```python
from build123d import *

# Parameters (mm, degrees)
SKETCH1_R           = 19.05
BOSS_EXTRUDE1_DEPTH = 76.2
SKETCH2_R           = 17.78
CUT_EXTRUDE1_DEPTH  = 69.85
CUT_EXTRUDE2_DEPTH  = 69.85
BOSS_EXTRUDE2_START = 6.35
SKETCH4_R           = 43.18
SKETCH4_R_2         = 17.78
BOSS_EXTRUDE2_DEPTH = 6.35
SKETCH5_R           = 12.7
BOSS_EXTRUDE3_DEPTH = 10.16
FILLET1_R           = 2.54
CHAMFER1_SIZE       = 2.54


with BuildPart() as part:
    # Sketch1 → Boss-Extrude1 (new body)
    with BuildSketch(Plane.XY):
        with Locations(Location((0, 0, 0), (0, 0, 180))):
            Circle(SKETCH1_R)
    extrude(amount=BOSS_EXTRUDE1_DEPTH)

    # Sketch2 → Cut-Extrude1 (cut)
    with BuildSketch(Plane.XY.offset(76.2)):
        Circle(SKETCH2_R)
    extrude(amount=-CUT_EXTRUDE1_DEPTH, mode=Mode.SUBTRACT)

    # Sketch3 → Cut-Extrude2 (cut)
    with BuildSketch(Plane.XY.offset(76.2)):
        with BuildLine():
            Line((-17.494221189, 3.175), (-18.783553311, 3.175))
            ThreePointArc((-18.783553311, 3.175), (-19.05, 0), (-18.783553311, -3.175))
            Line((-18.783553311, -3.175), (-17.494221189, -3.175))
            ThreePointArc((-17.494221189, -3.175), (-17.78, 0), (-17.494221189, 3.175))
        make_face()
        with BuildLine():
            ThreePointArc((19.05, 0), (18.983271459, 1.593080258), (18.783553311, 3.175))
            Line((18.783553311, 3.175), (17.494221189, 3.175))
            ThreePointArc((17.494221189, 3.175), (17.708411176, 1.593917699), (17.78, 0))
            ThreePointArc((17.78, 0), (17.708411176, -1.593917699), (17.494221189, -3.175))
            Line((17.494221189, -3.175), (18.783553311, -3.175))
            ThreePointArc((18.783553311, -3.175), (18.983271459, -1.593080258), (19.05, 0))
        make_face()
        with BuildLine():
            ThreePointArc((3.175, 18.783553311), (0, 19.05), (-3.175, 18.783553311))
            Line((-3.175, 18.783553311), (-3.175, 17.494221189))
            ThreePointArc((-3.175, 17.494221189), (0, 17.78), (3.175, 17.494221189))
            Line((3.175, 17.494221189), (3.175, 18.783553311))
        make_face()
        with BuildLine():
            Line((-3.175, -17.494221189), (-3.175, -18.783553311))
            ThreePointArc((-3.175, -18.783553311), (0, -19.05), (3.175, -18.783553311))
            Line((3.175, -18.783553311), (3.175, -17.494221189))
            ThreePointArc((3.175, -17.494221189), (0, -17.78), (-3.175, -17.494221189))
        make_face()
    extrude(amount=-CUT_EXTRUDE2_DEPTH, mode=Mode.SUBTRACT)

    # Sketch4 → Boss-Extrude2 (add)
    with BuildSketch(Plane.XY.offset(76.2).offset(BOSS_EXTRUDE2_START)):
        Circle(SKETCH4_R)
        Circle(SKETCH4_R_2, mode=Mode.SUBTRACT)
    extrude(amount=-BOSS_EXTRUDE2_DEPTH)

    # Sketch5 → Boss-Extrude3 (add)
    with BuildSketch(Plane(origin=(0, 0, 0), x_dir=(-1, 0, 0), z_dir=(0, 0, -1))):
        with Locations(Location((0, 0, 0), (0, 0, 180))):
            Circle(SKETCH5_R)
    extrude(amount=BOSS_EXTRUDE3_DEPTH)

    # Fillet1
    fillet1_edges = [part.edges().sort_by_distance(p)[0] for p in [
        (19.05, 0, 0),
        (-43.18, 0, 76.2),
        (-12.7, 0, -10.16),
    ]]
    fillet(fillet1_edges, radius=FILLET1_R)

    # Chamfer1
    # the kernel refuses this chamfer: 2.54 mm, written as the material it adds along each edge
    with BuildSketch(Plane(origin=(0, 0, 76.2), x_dir=(-0.9846344295499855, 0.1746282913641848, 0), z_dir=(0.1746282913641848, 0.9846344295499855, 0))) as chamfer1_piece_1_section:
        Polygon((19.05 + CHAMFER1_SIZE, 0), (19.05, -CHAMFER1_SIZE), (19.05, 0), align=None)
    chamfer1_piece_1 = revolve(axis=Axis((0, 0, 76.2), (0, 0, 1)), revolution_arc=110.114055389, mode=Mode.PRIVATE)
    chamfer1_piece_1 = split(chamfer1_piece_1, bisect_by=Plane(origin=(-19.847264072, 3.175, 75.490542074), z_dir=(0, 1, 0)), keep=Keep.TOP, mode=Mode.PRIVATE)
    add(chamfer1_piece_1)
    with BuildSketch(Plane(origin=(0, 0, 76.2), x_dir=(-0.9846344295499855, 0.1746282913641848, 0), z_dir=(0.1746282913641848, 0.9846344295499855, 0))) as chamfer1_piece_2_section:
        Polygon((19.05 + CHAMFER1_SIZE, 0), (19.05, -CHAMFER1_SIZE), (19.05, 0), align=None)
    chamfer1_piece_2 = revolve(axis=Axis((0, 0, 76.2), (0, 0, 1)), revolution_arc=110.114055389, mode=Mode.PRIVATE)
    chamfer1_piece_2 = split(chamfer1_piece_2, bisect_by=Plane(origin=(-14.346148442, -3.175, 74.961482306), z_dir=(0, -1, 0)), keep=Keep.TOP, mode=Mode.PRIVATE)
    chamfer1_piece_2 = split(chamfer1_piece_2, bisect_by=Plane(origin=(-3.175, -14.346148442, 74.961482306), z_dir=(-1, 0, 0)), keep=Keep.TOP, mode=Mode.PRIVATE)
    add(chamfer1_piece_2)
    with BuildSketch(Plane(origin=(0, 0, 76.2), x_dir=(-0.9846344295499855, 0.1746282913641848, 0), z_dir=(0.1746282913641848, 0.9846344295499855, 0))) as chamfer1_piece_3_section:
        Polygon((19.05 + CHAMFER1_SIZE, 0), (19.05, -CHAMFER1_SIZE), (19.05, 0), align=None)
    chamfer1_piece_3 = revolve(axis=Axis((0, 0, 76.2), (0, 0, 1)), revolution_arc=110.114055389, mode=Mode.PRIVATE)
    chamfer1_piece_3 = split(chamfer1_piece_3, bisect_by=Plane(origin=(3.175, -19.847263843, 75.490541907), z_dir=(1, 0, 0)), keep=Keep.TOP, mode=Mode.PRIVATE)
    add(chamfer1_piece_3)
    with BuildSketch(Plane(origin=(0, 0, 76.2), x_dir=(0.9846344295499821, -0.1746282913642033, 0), z_dir=(-0.1746282913642033, -0.9846344295499821, 0))) as chamfer1_piece_4_section:
        Polygon((19.05 + CHAMFER1_SIZE, 0), (19.05, -CHAMFER1_SIZE), (19.05, 0), align=None)
    chamfer1_piece_4 = revolve(axis=Axis((0, 0, 76.2), (0, 0, 1)), revolution_arc=110.114055389, mode=Mode.PRIVATE)
    chamfer1_piece_4 = split(chamfer1_piece_4, bisect_by=Plane(origin=(19.847264072, -3.175, 75.490542074), z_dir=(0, -1, 0)), keep=Keep.TOP, mode=Mode.PRIVATE)
    add(chamfer1_piece_4)
    with BuildSketch(Plane(origin=(0, 0, 76.2), x_dir=(0.9846344295499821, -0.1746282913642033, 0), z_dir=(-0.1746282913642033, -0.9846344295499821, 0))) as chamfer1_piece_5_section:
        Polygon((19.05 + CHAMFER1_SIZE, 0), (19.05, -CHAMFER1_SIZE), (19.05, 0), align=None)
    chamfer1_piece_5 = revolve(axis=Axis((0, 0, 76.2), (0, 0, 1)), revolution_arc=110.114055389, mode=Mode.PRIVATE)
    chamfer1_piece_5 = split(chamfer1_piece_5, bisect_by=Plane(origin=(14.346148442, 3.175, 74.961482306), z_dir=(0, 1, 0)), keep=Keep.TOP, mode=Mode.PRIVATE)
    chamfer1_piece_5 = split(chamfer1_piece_5, bisect_by=Plane(origin=(3.175, 14.346148442, 74.961482306), z_dir=(1, 0, 0)), keep=Keep.TOP, mode=Mode.PRIVATE)
    add(chamfer1_piece_5)
    with BuildSketch(Plane(origin=(0, 0, 76.2), x_dir=(0.9846344295499821, -0.1746282913642033, 0), z_dir=(-0.1746282913642033, -0.9846344295499821, 0))) as chamfer1_piece_6_section:
        Polygon((19.05 + CHAMFER1_SIZE, 0), (19.05, -CHAMFER1_SIZE), (19.05, 0), align=None)
    chamfer1_piece_6 = revolve(axis=Axis((0, 0, 76.2), (0, 0, 1)), revolution_arc=110.114055389, mode=Mode.PRIVATE)
    chamfer1_piece_6 = split(chamfer1_piece_6, bisect_by=Plane(origin=(-3.175, 19.847263843, 75.490541907), z_dir=(-1, 0, 0)), keep=Keep.TOP, mode=Mode.PRIVATE)
    add(chamfer1_piece_6)
    with BuildSketch(Plane(origin=(0, 0, 76.2), x_dir=(0.1746282913641894, 0.9846344295499847, 0), z_dir=(0.9846344295499847, -0.1746282913641894, 0))) as chamfer1_piece_7_section:
        Polygon((19.05 + CHAMFER1_SIZE, 0), (19.05, -CHAMFER1_SIZE), (19.05, 0), align=None)
    chamfer1_piece_7 = revolve(axis=Axis((0, 0, 76.2), (0, 0, 1)), revolution_arc=110.114055389, mode=Mode.PRIVATE)
    chamfer1_piece_7 = split(chamfer1_piece_7, bisect_by=Plane(origin=(3.175, 19.847264072, 75.490542074), z_dir=(1, 0, 0)), keep=Keep.TOP, mode=Mode.PRIVATE)
    add(chamfer1_piece_7)
    with BuildSketch(Plane(origin=(0, 0, 76.2), x_dir=(0.1746282913641894, 0.9846344295499847, 0), z_dir=(0.9846344295499847, -0.1746282913641894, 0))) as chamfer1_piece_8_section:
        Polygon((19.05 + CHAMFER1_SIZE, 0), (19.05, -CHAMFER1_SIZE), (19.05, 0), align=None)
    chamfer1_piece_8 = revolve(axis=Axis((0, 0, 76.2), (0, 0, 1)), revolution_arc=110.114055389, mode=Mode.PRIVATE)
    chamfer1_piece_8 = split(chamfer1_piece_8, bisect_by=Plane(origin=(-3.175, 14.346148442, 74.961482306), z_dir=(-1, 0, 0)), keep=Keep.TOP, mode=Mode.PRIVATE)
    chamfer1_piece_8 = split(chamfer1_piece_8, bisect_by=Plane(origin=(-14.346148442, 3.175, 74.961482306), z_dir=(0, 1, 0)), keep=Keep.TOP, mode=Mode.PRIVATE)
    add(chamfer1_piece_8)
    with BuildSketch(Plane(origin=(0, 0, 76.2), x_dir=(0.1746282913641894, 0.9846344295499847, 0), z_dir=(0.9846344295499847, -0.1746282913641894, 0))) as chamfer1_piece_9_section:
        Polygon((19.05 + CHAMFER1_SIZE, 0), (19.05, -CHAMFER1_SIZE), (19.05, 0), align=None)
    chamfer1_piece_9 = revolve(axis=Axis((0, 0, 76.2), (0, 0, 1)), revolution_arc=110.114055389, mode=Mode.PRIVATE)
    chamfer1_piece_9 = split(chamfer1_piece_9, bisect_by=Plane(origin=(-19.847263843, -3.175, 75.490541907), z_dir=(0, -1, 0)), keep=Keep.TOP, mode=Mode.PRIVATE)
    add(chamfer1_piece_9)
    with BuildSketch(Plane(origin=(0, 0, 76.2), x_dir=(-0.1746282913641849, -0.9846344295499855, 0), z_dir=(-0.9846344295499855, 0.1746282913641849, 0))) as chamfer1_piece_10_section:
        Polygon((19.05 + CHAMFER1_SIZE, 0), (19.05, -CHAMFER1_SIZE), (19.05, 0), align=None)
    chamfer1_piece_10 = revolve(axis=Axis((0, 0, 76.2), (0, 0, 1)), revolution_arc=110.114055389, mode=Mode.PRIVATE)
    chamfer1_piece_10 = split(chamfer1_piece_10, bisect_by=Plane(origin=(-3.175, -19.847264072, 75.490542074), z_dir=(-1, 0, 0)), keep=Keep.TOP, mode=Mode.PRIVATE)
    add(chamfer1_piece_10)
    with BuildSketch(Plane(origin=(0, 0, 76.2), x_dir=(-0.1746282913641849, -0.9846344295499855, 0), z_dir=(-0.9846344295499855, 0.1746282913641849, 0))) as chamfer1_piece_11_section:
        Polygon((19.05 + CHAMFER1_SIZE, 0), (19.05, -CHAMFER1_SIZE), (19.05, 0), align=None)
    chamfer1_piece_11 = revolve(axis=Axis((0, 0, 76.2), (0, 0, 1)), revolution_arc=110.114055389, mode=Mode.PRIVATE)
    chamfer1_piece_11 = split(chamfer1_piece_11, bisect_by=Plane(origin=(3.175, -14.346148442, 74.961482306), z_dir=(1, 0, 0)), keep=Keep.TOP, mode=Mode.PRIVATE)
    chamfer1_piece_11 = split(chamfer1_piece_11, bisect_by=Plane(origin=(14.346148442, -3.175, 74.961482306), z_dir=(0, -1, 0)), keep=Keep.TOP, mode=Mode.PRIVATE)
    add(chamfer1_piece_11)
    with BuildSketch(Plane(origin=(0, 0, 76.2), x_dir=(-0.1746282913641849, -0.9846344295499855, 0), z_dir=(-0.9846344295499855, 0.1746282913641849, 0))) as chamfer1_piece_12_section:
        Polygon((19.05 + CHAMFER1_SIZE, 0), (19.05, -CHAMFER1_SIZE), (19.05, 0), align=None)
    chamfer1_piece_12 = revolve(axis=Axis((0, 0, 76.2), (0, 0, 1)), revolution_arc=110.114055389, mode=Mode.PRIVATE)
    chamfer1_piece_12 = split(chamfer1_piece_12, bisect_by=Plane(origin=(19.847263843, 3.175, 75.490541907), z_dir=(0, 1, 0)), keep=Keep.TOP, mode=Mode.PRIVATE)
    add(chamfer1_piece_12)


solid = part.part
```
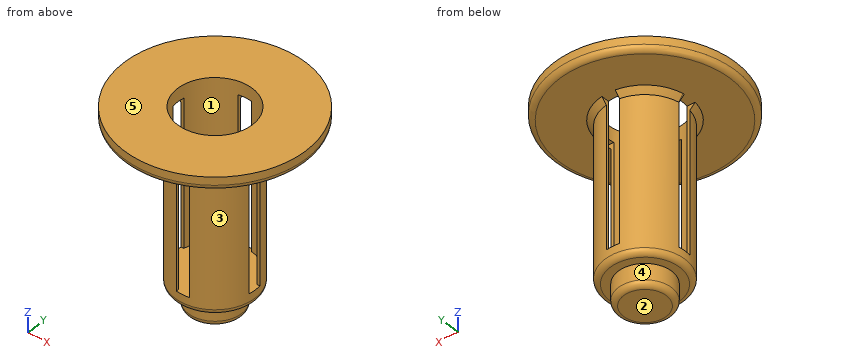
Verification items for the finished model (mm, model axes). Face numbers are marked on the shaded views. A direction names the side the tool comes from. Give positions to 0.01 mm unless a question says otherwise; leave off trailing zeros. Loops run counter-clockwise (first coordinate to the right, second up) from the corner with the lowest first, then second, coordinate; pieces in that order, holes last.
1. Thickness scan on line 1 (X direction, y = -5, z = 6.5); line 2 (Z direction, x = 18, y = 36); line 3 (Y direction, x = -10.5, z = 36.5). Record the ranges inside material, lowest first.
2. Set-up check for the marked faces 4 and 5: record each of +Z, -Z, +X, -X, +Y, -Y from which the full face is reachable in a straight line by a thin tool's end or side.
3. Section check A-A, the plane x = 0. Enter the section's corners in (y, z).
4. Mould release check, pull along Y, two halves, no side actions. Record for the marked faces 1, 2 and 3: released by +Y, released by -Y, zero draft, split by the parting line, or undercut.
5. Section check C-C, the plane z = 17. Enter the section's corners in (x, y) (3 decimals).
6. Go/stop test with flat-tipped pins: pin 1 Ø3 at (x, y) = (33, 16) entering from -Z; pin 2 Ø6 at (x, z) = (6, 50) entering from -Y; pin 3 Ø4 at (y, z) = (19, 53.5) entering from +X. Record where each tip stops, or that it passes through.
Geometry says:
1. line 1: x = -18.38 to -17.06, 17.06 to 18.38
1. line 2: z = 76.2 to 82.55
1. line 3: y = -15.9 to -14.35, 14.35 to 15.9
2. face 4: -Z
2. face 5: +Z, +X, -X, +Y, -Y
3. outline: (-43.18, 78.74) arc R2.54 ccw to (-40.64, 76.2) - (-17.78, 76.2) - (-17.78, 82.55) - (-43.18, 82.55) - close; (-19.05, 2.54) arc R2.54 ccw to (-16.51, 0) - (-12.7, 0) - (-12.7, -7.62) arc R2.54 ccw to (-10.16, -10.16) - (10.16, -10.16) arc R2.54 ccw to (12.7, -7.62) - (12.7, 0) - (16.51, 0) arc R2.54 ccw to (19.05, 2.54) - (19.05, 6.35) - (-19.05, 6.35) - close; (17.78, 76.2) - (40.64, 76.2) arc R2.54 ccw to (43.18, 78.74) - (43.18, 82.55) - (17.78, 82.55) - close
4. face 1: undercut
4. face 2: zero draft
4. face 3: split by the parting line
5. outline: (-18.784, -3.175) arc R19.05 ccw to (-3.175, -18.784) - (-3.175, -17.494) arc R17.78 cw to (-17.494, -3.175) - close; (-18.784, 3.175) - (-17.494, 3.175) arc R17.78 cw to (-3.175, 17.494) - (-3.175, 18.784) arc R19.05 ccw to start; (3.175, -18.784) arc R19.05 ccw to (18.784, -3.175) - (17.494, -3.175) arc R17.78 cw to (3.175, -17.494) - close; (3.175, 17.494) arc R17.78 cw to (17.494, 3.175) - (18.784, 3.175) arc R19.05 ccw to (3.175, 18.784) - close
6. pin 1: stops at z = 76.2
6. pin 2: stops at y = -18.78
6. pin 3: stops at x = 8.6
